Input: dimensioned drawing with shaded views. Units: mm. Origin: part minimum x, y, z. A direction names the side the tool comes from. Give positions to 0.01 mm unless a question says otherwise; leave off trailing zeros. Write each loop counter-clockwise with the first axis right and the second up, starting at its lowest first coordinate (ties: lowest second). Pieces come first, ordered by that corner, then holes. Notation, with made-up numbers: (10, 89) - (55, 89) arc R22 ccw to (55, 117) - close; hole circle Ø2 at (-12, -29). An arc over 180 degrees is marked (long way). Answer as a JSON object with one key per item and string values. Group by question number.
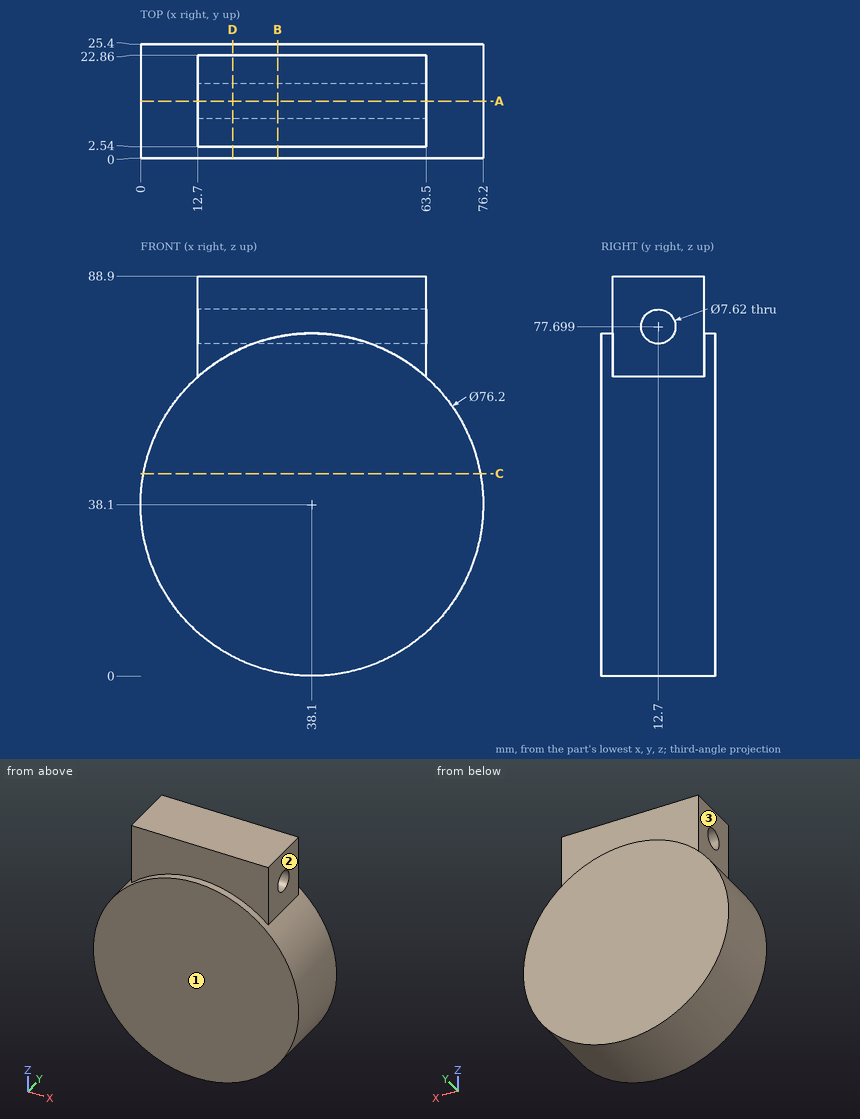
Q1. Section C-C on z = 45. Return the cut outline in (x, y), then the cut area to 3 significant figures.
Q2. Ray query, probe 1 along Z at (x, y) = (28, 12.7); probe 2 along Z at (x, y) = (24.5, 12.7); probe 3 along X at (y, z) = (19.5, 66.5). Return the intervals inside material, ascending. Write a range as [from, to].
Q3. First-contact query: pin 1 Ø6.5 at (x, z) = (51, 79.5) entering from -Y; pin 2 Ø2 at (y, z) = (6, 28) entering from -X; pin 3 Ø5 at (y, z) = (2.5, 24) entering from -X. Flat tips, straight axial feed; report the tip coordinate or a pass-through.
Q4. Section D-D on x = 20.5. Return the cut outline in (y, z), then the cut area to 3 significant figures.
Q5. Section A-A on y = 12.7. Return the cut outline in (x, z).
Q6. Section B-B on x = 30.5. Return the cut outline in (y, z), then the cut area to 3 significant figures.
Q7. Reachability of the marked faces 1, 2 and 3 from +Z, -Z, +X, -X, +Y, -Y: full face, straight path, thin tool, end or side. Return the list, or none.
Taken from the geometry:
{
 "1": {"outline": "(0.63, 0) - (75.57, 0) - (75.57, 25.4) - (0.63, 25.4) - close", "area": "1,900 mm²"},
 "2": {"probe 1": "z = [1.36, 73.89], [81.51, 88.9]", "probe 2": "z = [2.51, 73.89], [81.51, 88.9]", "probe 3": "x = [12.7, 63.5]"},
 "3": {"pin 1": "stops at y = 2.54", "pin 2": "stops at x = 1.1", "pin 3": "stops at x = 1.81"},
 "4": {"outline": "(0, 4.31) - (25.4, 4.31) - (25.4, 71.89) - (22.86, 71.89) - (22.86, 88.9) - (2.54, 88.9) - (2.54, 71.89) - (0, 71.89) - close; hole circle Ø7.62 at (12.7, 77.7)", "area": "2,020 mm²"},
 "5": {"outline": "(12.7, 66.5) arc R38.1 ccw (long way) to (63.5, 66.5) - (63.5, 73.89) - (12.7, 73.89) - close; (12.7, 81.51) - (63.5, 81.51) - (63.5, 88.9) - (12.7, 88.9) - close"},
 "6": {"outline": "(0, 0.77) - (25.4, 0.77) - (25.4, 75.43) - (22.86, 75.43) - (22.86, 88.9) - (2.54, 88.9) - (2.54, 75.43) - (0, 75.43) - close; hole circle Ø7.62 at (12.7, 77.7)", "area": "2,120 mm²"},
 "7": {"face 1": "+Z, -Z, +X, -X, -Y", "face 2": "+Z, +X, +Y, -Y", "face 3": "+Z, -X, +Y, -Y"}
}
